Design review of the part shown in the three views and the two pictorial views. Dimensions are in mm from the part's minimum x, y and z. A direction names the side the tool comes from. Round coordinates to 2 decimals unless told otherwise and drop trailing zeros. Use CSV: the item, a comma, the result in double quotes.
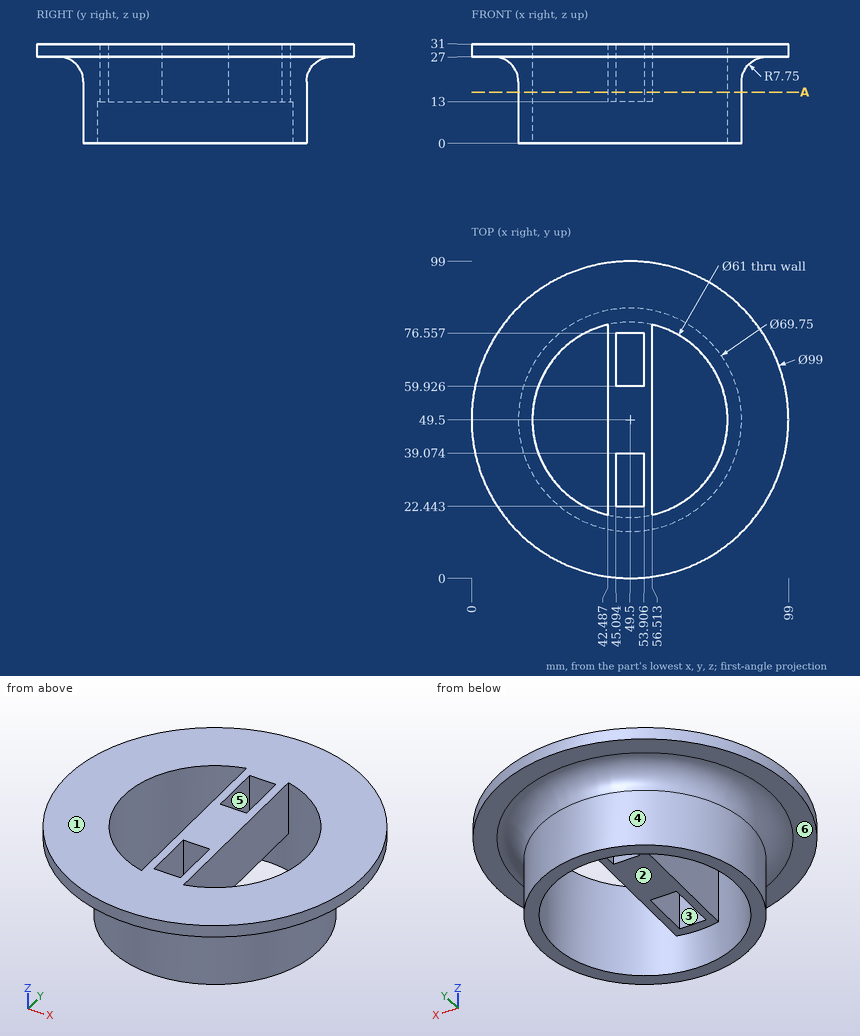
1) For the marked faces 1, 2 and 3, list the 3-axis set-ups (+Z, -Z, +X, -X, +Y, -Y) from which the entire face can be reached by the end or side of a thin tool; tool diameter is ignored.
Data:
face 1,"+Z, +X, -X, +Y, -Y"
face 2,"-Z"
face 3,"+Z, -Z"
2) We need section A-A (z = 16). Give the number of separate pieces and of enclosed holes in the cut face, then the cut area to 3 significant figures.
Data:
separate pieces,"1"
enclosed holes,"4"
area,"1,450 mm2"
3) To check wall thickness, follow L1, parallel to Y at x = 49.5, z = 9.5 (1 decimal); L2, parallel to X at y = 26, z = 23.5 (1 decimal); L3, parallel to X at y = 75, z = 19 (1 decimal). State the ranges of each line that lie inside material, in increasing order. Write a range as from..to.
Data:
L1,"y = 14.6..19, 80..84.4"
L2,"x = 22..30.1, 42.5..45.1, 53.9..56.5, 68.9..77"
L3,"x = 25.7..32.8, 42.5..45.1, 53.9..56.5, 66.2..73.3"
4) The part is to be moulded in two halves that separate along Y. For the marked faces 4, 5 and 6, say which applies: +Y half, -Y half, draft (parallel to the pull), parting line (faces both ways), or undercut.
Data:
face 4,"parting line"
face 5,"undercut"
face 6,"draft"
5) Insertion check: pin 1 Ø7 at (x, z) = (49.5, 22.5) entering from +Y (1 decimal); pin 2 Ø2 at (x, y) = (12, 77) entering from -Z; pin 3 Ø18.5 at (y, z) = (64.5, 26) entering from +X. Each pin has a flat end and moves straight along its axis. Give the tip position at first contact, or say it passes through.
Data:
pin 1,"stops at y = 88.3"
pin 2,"stops at z = 27"
pin 3,"stops at x = 98.66"
